```python
from build123d import *

# Parameters (mm, degrees)
F0_R     = 11.1125
F1_DEPTH = 1.5875
F2_R     = 6.985
F3_DEPTH = 1.27
F4_R     = 4.0005
F4_R_2   = 2.9845
F5_DEPTH = 2.0955


with BuildPart() as f1:
    # F0 (on Top) → F1 (new body)
    with BuildSketch(Plane.XY):
        Circle(F0_R)
    extrude(amount=F1_DEPTH)

    # F2 (on face) → F3 (join)
    with BuildSketch(Plane.XY.offset(1.5875)):
        Circle(F2_R)
    extrude(amount=F3_DEPTH)

    # F4 (on face) → F5 (join)
    with BuildSketch(Plane.XY.offset(2.8575)):
        Circle(F4_R)
        Circle(F4_R_2, mode=Mode.SUBTRACT)
    extrude(amount=F5_DEPTH)


solid = f1.part
```
Geometry: final body of the model. Coordinates: model frame, mm. A direction names the side the tool comes from. Coordinates: 2 decimals unless noted, no trailing zeros. Order: outer loops, then holes, each group sorted by start corner. A loop starts at its lowest first (then second) coordinate and runs counter-clockwise, first axis right, second up. Notation, with made-up numbers: (82.5, -23.75) -> (141.5, -23.75) arc R11 ccw to (141.5, -13.75) -> close; hole circle Ø8 at (48.25, 8.25). An arc over 180 degrees is marked (long way). Write each question's results on one line, items separated by ' | '. Start each with the question number.
1) Mould query, pull axis X, two halves, no side actions, for faces 3 (the cylindrical face through (-0.9, -3.9, 3.9)), 4 (the flat face through (-2, -3, 4.953)), 5 (the cylindrical face through (-0.647, -2.914, 3.891)). Classes: released by +X, released by -X, zero draft, split by the parting line, or undercut.
2) Set-up query: faces 1 (the cylindrical face through (10.6, 3.34, 0.78)), 2 (the cylindrical face through (-0.909, 6.926, 2.214)). Return all of +Z, -Z, +X, -X, +Y, -Y with unobstructed straight access to the full face (end or side cutting, diameter ignored); none if empty.
3) Material intervals for line 1 along Y through (x, z) = (0, 3.95); line 2 along Z through (x, y) = (3, -6.5); line 3 along Z through (x, y) = (-5, -2.5), sorted ascending.
4) Cut plane A-A, the plane x = 0. Output: boundary loops of the cut face in (y, z) (1 decimal).
5) Cut plane C-C, the plane z = 4.55. Output: boundary loops of the cut face in (x, y).
6) First-contact query: pin 1 (4 mm diameter, centred on x = 7.5, y = 8.5, fed in from +Z); pin 2 (11 mm diameter, centred on x = -0.5, y = -2, fed in from +Z); pin 3 (3 mm diameter, centred on x = 3, y = 5.5, fed in from +Z). Flat tips, straight axial feed; report the tip coordinate or a pass-through.
7) Cut plane D-D, the plane y = 6. Output: boundary loops of the cut face in (x, z), and give its area (3 significant figures).
Checks:
1) face 3: split by the parting line | face 4: zero draft | face 5: undercut
2) face 1: +Z, -Z | face 2: +Z
3) line 1: -4 to -2.98, 2.98 to 4 | line 2: 0 to 1.59 | line 3: 0 to 2.86
4) outline: (-11.1, 0) -> (11.1, 0) -> (11.1, 1.6) -> (7, 1.6) -> (7, 2.9) -> (4, 2.9) -> (4, 5) -> (3, 5) -> (3, 2.9) -> (-3, 2.9) -> (-3, 5) -> (-4, 5) -> (-4, 2.9) -> (-7, 2.9) -> (-7, 1.6) -> (-11.1, 1.6) -> close
5) outline: circle Ø8 at (0, 0); hole circle Ø5.97 at (0, 0)
6) pin 1: z = 1.59 | pin 2: z = 4.95 | pin 3: z = 2.86
7) outline: (-9.35, 0) -> (9.35, 0) -> (9.35, 1.59) -> (3.58, 1.59) -> (3.58, 2.86) -> (-3.58, 2.86) -> (-3.58, 1.59) -> (-9.35, 1.59) -> close | area: 38.8 mm^2
